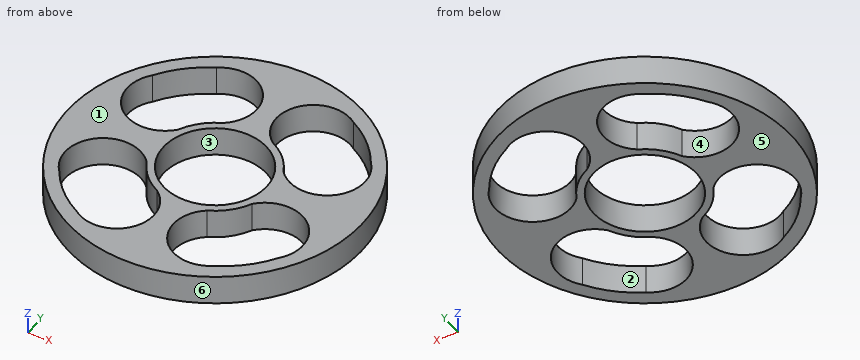
from build123d import *

# Parameters (mm, degrees)
F0_R     = 31.75
F0_R_2   = 11.1125
F1_DEPTH = 6.35
F3_DEPTH = 6.351


with BuildPart() as f1:
    # F0 (on Top) → F1 (new body)
    with BuildSketch(Plane.XY):
        Circle(F0_R)
        Circle(F0_R_2, mode=Mode.SUBTRACT)
    extrude(amount=F1_DEPTH)

    # F2 (on Top) → F3 (cut, through all)
    with BuildSketch(Plane.XY):
        with BuildLine():
            ThreePointArc((23.73958, 16.258981), (19.869054, 20.904466), (14.915959, 24.372658))
            ThreePointArc((14.915959, 24.372658), (3.730354, 22.660155), (5.442857, 11.47455))
            ThreePointArc((5.442857, 11.47455), (8.980256, 8.980256), (11.47455, 5.442857))
            ThreePointArc((11.47455, 5.442857), (23.015127, 4.718404), (23.73958, 16.258981))
        make_face()
        with BuildLine():
            ThreePointArc((14.915959, -24.372658), (19.869054, -20.904466), (23.73958, -16.258981))
            ThreePointArc((23.73958, -16.258981), (23.015127, -4.718404), (11.47455, -5.442857))
            ThreePointArc((11.47455, -5.442857), (8.980256, -8.980256), (5.442857, -11.47455))
            ThreePointArc((5.442857, -11.47455), (3.730354, -22.660155), (14.915959, -24.372658))
        make_face()
        with BuildLine():
            ThreePointArc((-5.442857, 11.47455), (-3.730354, 22.660155), (-14.915959, 24.372658))
            ThreePointArc((-14.915959, 24.372658), (-19.869054, 20.904466), (-23.73958, 16.258981))
            ThreePointArc((-23.73958, 16.258981), (-23.015127, 4.718404), (-11.47455, 5.442857))
            ThreePointArc((-11.47455, 5.442857), (-8.980256, 8.980256), (-5.442857, 11.47455))
        make_face()
        with BuildLine():
            ThreePointArc((-5.442857, -11.47455), (-8.980256, -8.980256), (-11.47455, -5.442857))
            ThreePointArc((-11.47455, -5.442857), (-23.015127, -4.718404), (-23.73958, -16.258981))
            ThreePointArc((-23.73958, -16.258981), (-19.869054, -20.904466), (-14.915959, -24.372658))
            ThreePointArc((-14.915959, -24.372658), (-3.730354, -22.660155), (-5.442857, -11.47455))
        make_face()
    extrude(amount=F3_DEPTH, mode=Mode.SUBTRACT)


solid = f1.part
Here's how the part is built. I have some questions about the finished solid (model axes, mm). Face numbers are marked on the shaded views. A direction names the side the tool comes from. Coordinates: 2 decimals unless noted, no trailing zeros. Order: outer loops, then holes, each group sorted by start corner. A loop starts at its lowest first (then second) coordinate and runs counter-clockwise, first axis right, second up. Notation, with made-up numbers: M -35,-18 L -24,-18 A16 cw -24,13 Z; hole C -11,22 d11. An arc over 180 degrees is marked long. Answer as CSV lines item,"result".
Item 1: If I drill on line 1 (Y direction, x = 0, z = 4.75); line 2 (X direction, y = 3.5, z = 5); line 3 (Y direction, x = 18, z = 3), over which ranges is the centre line in solid material (lowest first)?
Results found:
line 1,"-31.75 to -11.11, 11.11 to 31.75"
line 2,"-31.56 to -21.19, -14.03 to -10.55, 10.55 to 14.03, 21.19 to 31.56"
line 3,"-26.15 to -22.45, -2.68 to 2.68, 22.45 to 26.15"
Item 2: Imagine slicing it at A-A on y = 0. Write out the boundary of the cut face in (x, z).
Results found:
outline,"M -31.75,0 L -11.11,0 L -11.11,6.35 L -31.75,6.35 Z; M 11.11,0 L 31.75,0 L 31.75,6.35 L 11.11,6.35 Z"
Item 3: Imagine slicing it at C-C on z = 1. Give the number of separate pieces and of enclosed holes in the cut face, plus the area to 3 significant figures.
Results found:
separate pieces,"1"
enclosed holes,"5"
area,"1,290 mm2"
Item 4: We'd pull the mould along Y, two halves only. Please class the marked faces 3, 4, 5 and 6: +Y half, -Y half, draft (parallel to the pull), parting line (faces both ways), or undercut.
Results found:
face 3,"undercut"
face 4,"undercut"
face 5,"draft"
face 6,"parting line"
Item 5: For pin 1 (2 mm diameter, centred on y = -7.5, z = 2.5, fed in from +X), with a flat end and sliding along its axis, tell me the tip position at first contact or that it passes through.
Results found:
pin 1,"x = 31.08"
Item 6: Imagine slicing it at D-D on x = 7. Write out the boundary of the cut face in (y, z), plus the area to 3 significant figures.
Results found:
outline,"M -30.97,0 L -25.27,0 L -25.27,6.35 L -30.97,6.35 Z; M -10.6,0 L -8.63,0 L -8.63,6.35 L -10.6,6.35 Z; M 8.63,0 L 10.6,0 L 10.6,6.35 L 8.63,6.35 Z; M 25.27,0 L 30.97,0 L 30.97,6.35 L 25.27,6.35 Z"
area,"97.4 mm2"
Item 7: On a 3-axis mill with a long thin cutter (end or side, diameter ignored), from which of +Z, -Z, +X, -X, +Y, -Y can I reach the whole of each face in a straight line? I mean the marked faces 1 and 2. Say none if no direction works.
Results found:
face 1,"+Z, +X, -X, +Y, -Y"
face 2,"+Z, -Z"
